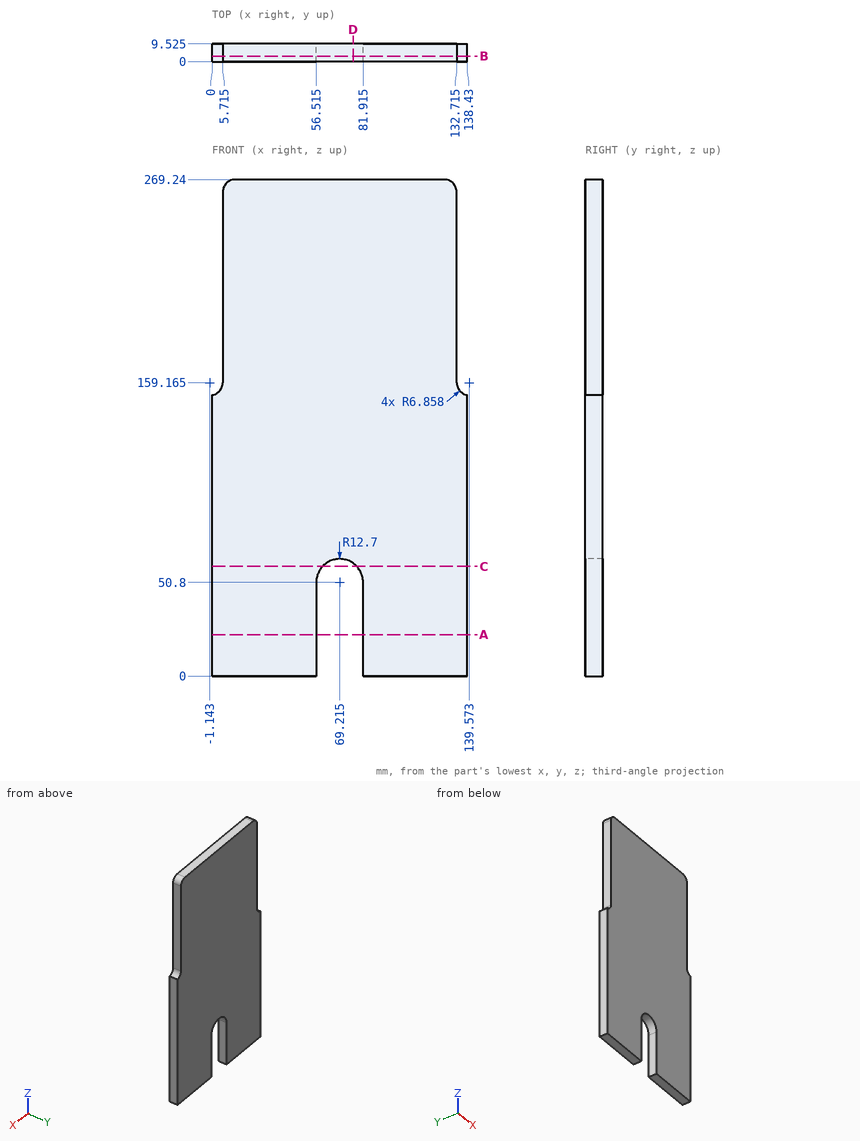
Part print with two shaded views. Sizes in mm from the minimum x, y, z corner. Give positions to 0.01 mm unless a question says otherwise; leave off trailing zeros. Order: outer loops, then holes, each group sorted by start corner. A loop starts at its lowest first (then second) coordinate and runs counter-clockwise, first axis right, second up.
1) Pin check, flat tips, straight feed: pin 1 (3 mm diameter, centred on y = 2.5, z = 191, fed in from +X) (3 decimals); pin 2 (5 mm diameter, centred on y = 6, z = 188.5, fed in from -X) (3 decimals). Stop position of each tip, or through.
2) Saw through at C-C, the plane z = 59.5. Write the cut outline in (x, y) (1 decimal), then the cut area to 3 significant figures.
3) Saw through at D-D, the plane x = 76.5. Write the cut outline in (y, z) (1 decimal).
4) Saw through at A-A, the plane z = 22.5. Write the cut outline in (x, y) (1 decimal), then the cut area to 3 significant figures.
5) Wall check: probe 1 along X at (y, z) = (2, 18.5) (1 decimal); probe 2 along X at (y, z) = (8, 225.5) (1 decimal); probe 3 along Z at (x, y) = (68, 1.75). Give the ranges that are in metal, low to high.
6) Saw through at B-B, the plane y = 3. Write the cut outline in (x, z) (1 decimal), then the cut area to 3 significant figures.
Computed:
1. pin 1: stops at x = 132.715
1. pin 2: stops at x = 5.715
2. outline: (0, 0) - (60, 0) - (60, 9.5) - (0, 9.5) - close; (78.5, 0) - (138.4, 0) - (138.4, 9.5) - (78.5, 9.5) - close
2. area: 1,140 mm2
3. outline: (0, 61.2) - (9.5, 61.2) - (9.5, 269.2) - (0, 269.2) - close
4. outline: (0, 0) - (56.5, 0) - (56.5, 9.5) - (0, 9.5) - close; (81.9, 0) - (138.4, 0) - (138.4, 9.5) - (81.9, 9.5) - close
4. area: 1,080 mm2
5. probe 1: x = 0 to 56.5, 81.9 to 138.4
5. probe 2: x = 5.7 to 132.7
5. probe 3: z = 63.44 to 269.24
6. outline: (0, 0) - (56.5, 0) - (56.5, 50.8) arc R12.7 cw to (81.9, 50.8) - (81.9, 0) - (138.4, 0) - (138.4, 152.4) arc R6.9 cw to (132.7, 159.2) - (132.7, 262.4) arc R6.9 ccw to (125.9, 269.2) - (12.6, 269.2) arc R6.9 ccw to (5.7, 262.4) - (5.7, 159.2) arc R6.9 cw to (0, 152.4) - close
6. area: 34,400 mm2
